The listing builds one solid part. Answer for the finished solid, in the listing's coordinates (mm). Face numbers are marked on the shaded views. A direction names the side the tool comes from. Give positions to 0.01 mm unless a question says otherwise; leave off trailing zeros. Loops run counter-clockwise (first coordinate to the right, second up) from the corner with the lowest first, then second, coordinate; pieces in that order, holes last. Notation, with made-up numbers: M -22,12.5 L -18,12.5 A13 cw -18,27.5 Z; hole C 12,32.5 d10. An arc over 180 degrees is marked long. One line per item, written item: value. Start each with the question number.
Q1. For the marked faces 5 and 6, determine the directions among +Z, -Z, +X, -X, +Y, -Y from which every point of the face is accessible in a straight line to the end or side of a thin tool.
Q2. The mould has two halves that part along X. Classify the marked faces 1, 2, 3 and 4: +X half, -X half, draft (parallel to the pull), parting line (faces both ways), or undercut.
Q3. A cutting plane is placed at B-B, the plane y = 0. Determine the outline of the cut face in (x, z).
Q4. A cutting plane is placed at A-A, the plane x = 3.5. Determine the outline of the cut face in (y, z).
Q5. A cutting plane is placed at C-C, the plane x = -23. Determine the outline of the cut face in (y, z), and give its area (3 significant figures).
Q6. Consider L1, parallel to Y at x = 0, z = 2.25; L2, parallel to X at y = -22, z = 2.2; L3, parallel to Y at x = 5, z = 3.55. Determine where each line is inside the solid, lowest interval first.
Q7. A cutting plane is placed at D-D, the plane y = 9.5. Determine the outline of the cut face in (x, z), and give its area (3 significant figures).
Q8. Flat-ended cylindrical pins translate along their axes: pin 1 (2.5 mm diameter, centred on x = 2, z = 3, fed in from -Y); pin 2 (2.5 mm diameter, centred on y = -23.5, z = 2.5, fed in from +X). Find the tip coordinate at first contact, or state that the pin passes through.
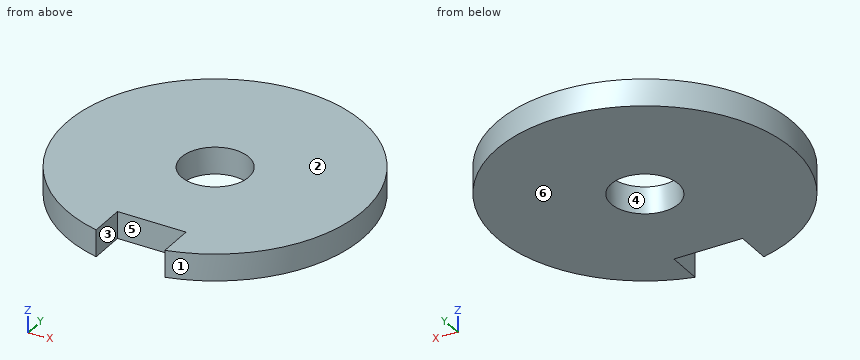
from build123d import *

# Parameters (mm, degrees)
F0_R     = 27.5
F1_DEPTH = 5
F2_R     = 6.25
F3_DEPTH = 25
F4_W     = 9.638923
F4_H     = 7.71114
F5_DEPTH = 5
F6_W     = 12.723378
F6_H     = 9.831702
F7_DEPTH = 25


with BuildPart() as f1:
    # F0 (on Top) → F1 (new body)
    with BuildSketch(Plane.XY):
        with Locations((-0.094615, 0.134945)):
            Circle(F0_R)
    extrude(amount=F1_DEPTH)

    # F2 (on face) → F3 (cut)
    with BuildSketch(Plane.XY.offset(5)):
        Circle(F2_R)
    extrude(amount=-F3_DEPTH, mode=Mode.SUBTRACT)

    # F4 (on face) → F5 (cut)
    with BuildSketch(Plane.XY.offset(5)):
        with Locations((0.578336, -24.772032)):
            Rectangle(F4_W, F4_H)
    extrude(amount=-F5_DEPTH, mode=Mode.SUBTRACT)

    # F6 (on face) → F7 (cut)
    with BuildSketch(Plane.XY.offset(5)):
        with Locations((-1e-06, -24.868422)):
            Rectangle(F6_W, F6_H)
    extrude(amount=-F7_DEPTH, mode=Mode.SUBTRACT)


solid = f1.part
Answer block:
1. face 5: +Z, -Z, -Y
1. face 6: -Z, +X, -X, +Y, -Y
2. face 1: parting line
2. face 2: draft
2. face 3: undercut
2. face 4: undercut
3. outline: M -27.59,0 L -6.25,0 L -6.25,5 L -27.59,5 Z; M 6.25,0 L 27.41,0 L 27.41,5 L 6.25,5 Z
4. outline: M -19.95,0 L -5.18,0 L -5.18,5 L -19.95,5 Z; M 5.18,0 L 27.4,0 L 27.4,5 L 5.18,5 Z
5. outline: M -15.08,0 L 15.35,0 L 15.35,5 L -15.08,5 Z
5. area: 152 mm^2
6. L1: -19.95 to -6.25, 6.25 to 27.63
6. L2: -16.41 to -6.36, 6.36 to 16.22
6. L3: -19.95 to -3.75, 3.75 to 27.16
7. outline: M -25.95,0 L 25.76,0 L 25.76,5 L -25.95,5 Z
7. area: 259 mm^2
8. pin 1: y = -19.95
8. pin 2: x = 15.88
